Check sheet for the modelled part. Datum: model origin and axes. Units: mm. A direction names the side the tool comes from. Give positions to 0.01 mm unless a question says otherwise; leave off trailing zeros. Write each loop counter-clockwise with the first axis right and the second up, starting at its lowest first coordinate (ties: lowest second). Pieces come first, ordered by that corner, then holes. Notation, with made-up numbers: M -33,-1 L 13,-1 A29 ccw 13,26 Z; hole C 53,-39.75 d6. An arc over 180 degrees is marked long. One line per item, written item: value. Start each with the question number.
from build123d import *

# Parameters (mm, degrees)
BOSS_EXTRUDE1_DEPTH = 25.4
CUT_EXTRUDE1_REACH  = 51.74
SKETCH3_R           = 3.3734375
CUT_EXTRUDE2_REACH  = 51.74
SKETCH4_R           = 3.3734375
SKETCH6_W           = 38.925
SKETCH6_H           = 64.325
SKETCH6_W_2         = 34.925
SKETCH6_H_2         = 60.325
BOSS_EXTRUDE4_DEPTH = 50.8
CUT_EXTRUDE3_DEPTH  = 5.08
CUT_EXTRUDE3_DRAFT  = -4.3
SKETCH9_W           = 34.925
SKETCH9_H           = 60.325
BOSS_EXTRUDE6_DEPTH = 3.175


with BuildPart() as part:
    # Sketch1 → Boss-Extrude1 (new body)
    with BuildSketch(Plane(origin=(0, 0, 0), x_dir=(1, 0, 0), z_dir=(0, 1, 0))):
        with BuildLine():
            Line((17.840314435, -9.593687765), (19.948512047, -3.517460899))
            Line((19.948512047, -3.517460899), (17.978896541, -3.170164544))
            ThreePointArc((17.978896541, -3.170164544), (-18.25625, 0), (17.978896541, 3.170164544))
            Line((17.978896541, 3.170164544), (19.948512047, 3.517460899))
            Line((19.948512047, 3.517460899), (17.840314435, 9.593687765))
            ThreePointArc((17.840314435, 9.593687765), (-20.25625, 0), (17.840314435, -9.593687765))
        make_face()
        with BuildLine():
            Line((30.744742589, 11.869086619), (17.840314435, 9.593687765))
            ThreePointArc((17.840314435, 9.593687765), (19.137110151, 6.63978005), (19.948512047, 3.517460899))
            Line((19.948512047, 3.517460899), (32.45557051, 5.722792755))
            Line((32.45557051, 5.722792755), (30.744742589, 11.869086619))
        make_face()
        with BuildLine():
            Line((32.45557051, -5.722792755), (19.948512047, -3.517460899))
            ThreePointArc((19.948512047, -3.517460899), (19.137110151, -6.63978005), (17.840314435, -9.593687765))
            Line((17.840314435, -9.593687765), (30.744742589, -11.869086619))
            Line((30.744742589, -11.869086619), (32.45557051, -5.722792755))
        make_face()
        with BuildLine():
            ThreePointArc((17.840314435, -9.593687765), (19.137110151, -6.63978005), (19.948512047, -3.517460899))
            Line((19.948512047, -3.517460899), (17.840314435, -9.593687765))
        make_face()
        with BuildLine():
            ThreePointArc((19.948512047, 3.517460899), (19.137110151, 6.63978005), (17.840314435, 9.593687765))
            Line((17.840314435, 9.593687765), (19.948512047, 3.517460899))
        make_face()
    extrude(amount=BOSS_EXTRUDE1_DEPTH)

    # Sketch3 → Cut-Extrude1 (cut, up to next)
    with BuildSketch(Plane(origin=(-1.102665928, 0, 6.253529232), x_dir=(0.984807753012208, 0, 0.17364817766693044), z_dir=(-0.17364817766693044, 0, 0.984807753012208)), mode=Mode.PRIVATE) as cut_extrude1_sk1:
        with Locations((25.988706128, 12.7)):
            Circle(SKETCH3_R)
    cut_extrude1_tool1 = extrude(cut_extrude1_sk1.sketch, amount=-CUT_EXTRUDE1_REACH, mode=Mode.PRIVATE) & part.part
    add(cut_extrude1_tool1.solids().sort_by_distance((24.491213, 12.7, 10.766421))[0], mode=Mode.SUBTRACT)

    # Sketch4 → Cut-Extrude2 (cut, up to next)
    with BuildSketch(Plane(origin=(-1.102665928, 0, -6.253529232), x_dir=(-0.984807753012208, 0, 0.17364817766693136), z_dir=(-0.17364817766693136, 0, -0.984807753012208)), mode=Mode.PRIVATE) as cut_extrude2_sk1:
        with Locations((-25.988706128, 12.7)):
            Circle(SKETCH4_R)
    cut_extrude2_tool1 = extrude(cut_extrude2_sk1.sketch, amount=-CUT_EXTRUDE2_REACH, mode=Mode.PRIVATE) & part.part
    add(cut_extrude2_tool1.solids().sort_by_distance((24.491213, 12.7, -10.766421))[0], mode=Mode.SUBTRACT)

    # Sketch6 → Boss-Extrude4 (add)
    with BuildSketch(Plane.XZ):
        with Locations((-37.71875, 0)):
            Rectangle(SKETCH6_W, SKETCH6_H)
        with Locations((-37.71875, 0)):
            Rectangle(SKETCH6_W_2, SKETCH6_H_2, mode=Mode.SUBTRACT)
    extrude(amount=-BOSS_EXTRUDE4_DEPTH)


with BuildPart() as cut_extrude3_tool:
    # Sketch8 → Cut-Extrude3 (with draft: the straight prism first)
    with BuildSketch(Plane(origin=(-1.102665928, 0, -6.253529232), x_dir=(-0.984807753012208, 0, 0.17364817766693136), z_dir=(-0.17364817766693136, 0, -0.984807753012208))):
        Polygon((-20.273706128, 9.400443212), (-20.273706128, 15.999556788), (-25.988706128, 19.299113577), (-31.703706128, 15.999556788), (-31.703706128, 9.400443212), (-25.988706128, 6.100886423), align=None)
    extrude(amount=-CUT_EXTRUDE3_DEPTH)
    # Cut-Extrude3: the draft: its side faces are tilted about the plane it starts from
    cut_extrude3_sides = [cut_extrude3_tool.faces().sort_by_distance(p)[0] for p in [
        (19.304103421, 12.7, -7.272609663),
        (22.118191575, 17.649335183, -7.76880933),
        (27.746367883, 17.649335183, -8.761208666),
        (30.560456038, 12.7, -9.257408333),
        (27.746367883, 7.750664817, -8.761208666),
        (22.118191575, 7.750664817, -7.76880933),
    ]]
    draft(cut_extrude3_sides, Plane(origin=(-1.102665928, 0, -6.253529232), x_dir=(-0.984807753012208, 0, 0.17364817766693136), z_dir=(-0.17364817766693136, 0, -0.984807753012208)), CUT_EXTRUDE3_DRAFT)


with BuildPart() as part_1:
    add(part.part)

    # Cut-Extrude3: cut by cut_extrude3_tool
    add(cut_extrude3_tool.part, mode=Mode.SUBTRACT)

    # Sketch9 → Boss-Extrude6 (add)
    with BuildSketch(Plane.XZ):
        with Locations((-37.71875, 0)):
            Rectangle(SKETCH9_W, SKETCH9_H)
    extrude(amount=-BOSS_EXTRUDE6_DEPTH)


solid = part_1.part
1) Gauge pin test, flat ends, axial feed: pin 1 (22.5 mm diameter, centred on x = 9.5, z = -12, fed in from +Y); pin 2 (10 mm diameter, centred on x = 19.5, y = 35, fed in from -Z). Record the tip position at first contact, or that the pin passes through.
2) Tool access check on faces 1 (the flat face through (14, 25.4, -12)), 2 (the flat face through (18.648, 12.522, -9.736)), 3 (the flat face through (19.483, 12.654, -7.34)). Record the directions out of +Z, -Z, +X, -X, +Y, -Y that give a thin tool (end or side, any length) a straight path to the whole face; none if there is none.
3) Cross-section at A-A (x = 0). Record the boundary of the cut face in (y, z), plus the area to 3 significant figures.
4) Cross-section at D-D (x = -23). Record the boundary of the cut face in (y, z) (1 decimal).
5) Cross-section at B-B (y = 33). Record the boundary of the cut face in (x, z).
6) Draft check along X on faces 4 (the cylindrical face through (-18.24, 12.52, 0.76)), 5 (the flat face through (-33, 0, 0)), 6 (the flat face through (31.6, 12.5, -8.8)). Enter one of: released by +X, released by -X, zero draft, split by the parting line, or undercut.
7) Cross-section at C-C (z = -24). Record the boundary of the cut face in (x, y) (3 decimals).
8) Material ranges on L1, parallel to Z at x = 0, y = 5.25; L2, parallel to X at y = 6, z = 28; L3, parallel to X at y = 22.5, z = -7.5, recorded low to high. Write a range as from..to.
Data:
1. pin 1: stops at y = 25.4
1. pin 2: passes through
2. face 1: +Z, -Z, +X, +Y
2. face 2: -Z, +Y, -Y
2. face 3: -Z
3. outline: M 0,-20.26 L 25.4,-20.26 L 25.4,-18.26 L 0,-18.26 Z; M 0,18.26 L 25.4,18.26 L 25.4,20.26 L 0,20.26 Z
3. area: 102 mm2
4. outline: M 0,-32.2 L 50.8,-32.2 L 50.8,-30.2 L 3.2,-30.2 L 3.2,30.2 L 50.8,30.2 L 50.8,32.2 L 0,32.2 Z
5. outline: M -57.18,-32.16 L -18.26,-32.16 L -18.26,32.16 L -57.18,32.16 Z; hole M -55.18,-30.16 L -20.26,-30.16 L -20.26,30.16 L -55.18,30.16 Z
6. face 4: undercut
6. face 5: zero draft
6. face 6: released by +X
7. outline: M -57.181,0 L -18.256,0 L -18.256,50.8 L -20.256,50.8 L -20.256,3.175 L -55.181,3.175 L -55.181,50.8 L -57.181,50.8 Z
8. L1: z = -20.26..-18.26, 18.26..20.26
8. L2: x = -57.18..-55.18, -20.26..-18.26
8. L3: x = -57.18..-55.18, -20.26..-16.64, 16.64..31.96
